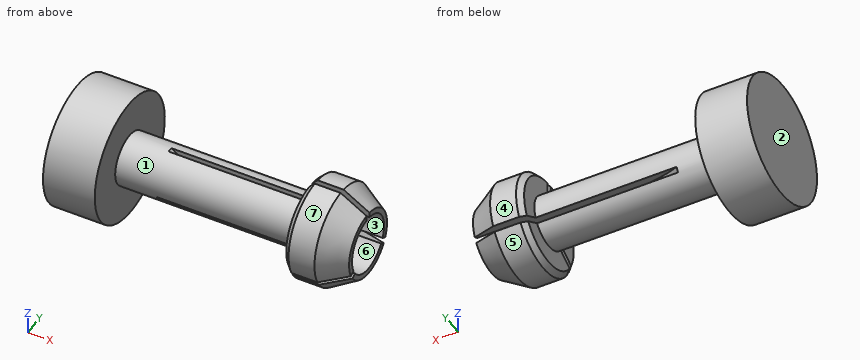
from build123d import *

# Parameters (mm, degrees)
F2_SIZE  = 1
F4_DEPTH = 0.5
F5_COUNT = 3


with BuildPart() as f1:
    # F0 (on Front) → F1 (revolve)
    with BuildSketch(Plane.XZ):
        Polygon((35, 5), (0, 5), (0, 12), (-10, 12), (-10, 0), (0, 0), (40, 0), (40, 5.5), (46, 5.5), (46, 6.5), (41, 9.5), (35, 9.5), align=None)
    revolve(axis=Axis((23.443235, 0, 0), (1, 0, 0)))

    # F2
    f2_edges = [f1.edges().sort_by_distance(p)[0] for p in [
        (35, 0, -9.5),
    ]]
    chamfer(f2_edges, length=F2_SIZE)


with BuildPart() as f4:
    # F3 (on Front) → F4 (new body, symmetric)
    with BuildSketch(Plane.XZ):
        with BuildLine():
            Line((55.388199, 40), (21, 40))
            ThreePointArc((21, 40), (1, 20), (21, 0))
            Line((21, 0), (55.388199, 0))
            Line((55.388199, 0), (55.388199, 40))
        make_face()
    extrude(amount=F4_DEPTH, both=True)


with BuildPart() as f5_1:
    # F5: instance of F4
    add(f4.part.rotate(Axis((62.455053, 0, 0), (1, 0, 0)), 1 * 360 / F5_COUNT))


with BuildPart() as f5_2:
    # F5: instance of F4
    add(f4.part.rotate(Axis((62.455053, 0, 0), (1, 0, 0)), 2 * 360 / F5_COUNT))


with BuildPart() as f1_1:
    add(f1.part)

    # F6: cut F4, F5_1, F5_2
    add(f4.part, mode=Mode.SUBTRACT)
    add(f5_1.part, mode=Mode.SUBTRACT)
    add(f5_2.part, mode=Mode.SUBTRACT)


solid = f1_1.part
For this review, take the finished solid that the model builds, in its own axes (mm). Face numbers are marked on the shaded views. A direction names the side the tool comes from. Coordinates: 2 decimals unless noted, no trailing zeros. Order: outer loops, then holes, each group sorted by start corner. A loop starts at its lowest first (then second) coordinate and runs counter-clockwise, first axis right, second up. Notation, with made-up numbers: (-19.75, -31) -> (8.25, -31) arc R31 ccw to (8.25, -4) -> close; hole circle Ø5 at (83, 5). An arc over 180 degrees is marked (long way). Return JSON: item names as keys, results as strings.
1. We need section A-A on x = 42. Write out the cut boundary in (y, z).
Answer block:
{"outline": "(-7.95, -4.01) -> (-4.99, -2.31) arc R5.5 cw to (-0.5, 5.48) -> (-0.5, 8.89) arc R8.9 ccw to start; (-7.45, -4.88) arc R8.9 ccw to (7.45, -4.88) -> (4.49, -3.17) arc R5.5 cw to (-4.49, -3.17) -> close; (0.5, 5.48) arc R5.5 cw to (4.99, -2.31) -> (7.95, -4.01) arc R8.9 ccw to (0.5, 8.89) -> close"}
2. For line 1 (Y direction, x = 41, z = 1.5); line 2 (Y direction, x = 27, z = 2); line 3 (Y direction, x = 14.5, z = 0), list the stretches that pass through material, from the lowest coordinate up. Write a range as from..to.
Answer block:
{"line 1": "-9.38..-5.29, 5.29..9.38", "line 2": "-4.58..-0.5, 0.5..4.58", "line 3": "-5..5"}
3. We need section D-D on z = 7.75. State how many separate pieces and enclosed holes the cut face has, and give its area (3 significant figures).
Answer block:
{"separate pieces": "3", "enclosed holes": "0", "area": "259 mm²"}
4. We need section C-C on y = -10.25. Write out the cut boundary in (x, z).
Answer block:
{"outline": "(-10, -6.24) -> (0, -6.24) -> (0, 6.24) -> (-10, 6.24) -> close"}
5. For pin 1 Ø2 at (x, z) = (30.5, -4.5) entering from +Y; pin 2 Ø1 at (x, z) = (10.5, 4.5) entering from -Y; pin 3 Ø12 at (y, z) = (-7.5, -4) entering from +X; pin 4 Ø3 at (x, z) = (29, 3.5) entering from -Y, all flat-tipped, find the tip position at first contact; note any pin that passes through.
Answer block:
{"pin 1": "y = 3.57", "pin 2": "y = -3", "pin 3": "x = 46", "pin 4": "y = -4.58"}
6. The part is to be moulded in two halves that separate along X. For the marked faces 1, 2 and 3, say which applies: +X half, -X half, draft (parallel to the pull), parting line (faces both ways), or undercut.
Answer block:
{"face 1": "undercut", "face 2": "-X half", "face 3": "draft"}
7. We need section B-B on x = 15.5. Write out the cut boundary in (y, z).
Answer block:
{"outline": "(-4.56, -2.05) -> (-0.92, 0.05) -> (-0.42, -0.82) -> (-4.06, -2.92) arc R5 ccw to (4.06, -2.92) -> (0.42, -0.82) -> (0.92, 0.05) -> (4.56, -2.05) arc R5 ccw to (0.5, 4.97) -> (0.5, 0.77) -> (-0.5, 0.77) -> (-0.5, 4.97) arc R5 ccw to start"}
8. Machinability: for the marked faces 4, 5, 6 and 7, which of the approach directions +Z, -Z, +X, -X, +Y, -Y give a long, thin tool a straight path to every point of the face, cutting with its end or side? Answer none if there is none.
Answer block:
{"face 4": "+X, +Y", "face 5": "-Z, +X", "face 6": "+X", "face 7": "+X, -Y"}
